Could you check a few things on this drawing? It's one solid part, dimensions in mm from its lowest x, y, z. Give positions to 0.01 mm unless a question says otherwise; leave off trailing zeros. Write each loop counter-clockwise with the first axis right and the second up, starting at its lowest first coordinate (ties: lowest second). Pieces come first, ordered by that corner, then holes. Notation, with made-up numbers: M 68.25,0.5 L 83.25,0.5 A13 cw 83.25,22.5 Z; hole C -8.75,54 d1. An arc over 180 degrees is marked long. Answer as CSV lines item,"result". Start each with the question number.
Q1. For pin 1 (8 mm diameter, centred on y = 5.5, z = 14, fed in from -X), with a flat end and sliding along its axis, tell me the tip position at first contact or that it passes through.
Q2. Suppose I cut it at A-A (z = 19). Write out the boundary of the cut face in (x, y) (1 decimal), then the cut area to 3 significant figures.
Q3. If I drill on line 1 along X through (y, z) = (37.5, 12.5); line 2 along X through (y, z) = (28.5, 12) (1 decimal); line 3 along Y through (x, z) = (16, 18.75), over which ranges is the centre line in solid material (lowest first)?
Q4. Suppose I cut it at B-B (x = 190). Write out the boundary of the cut face in (y, z).
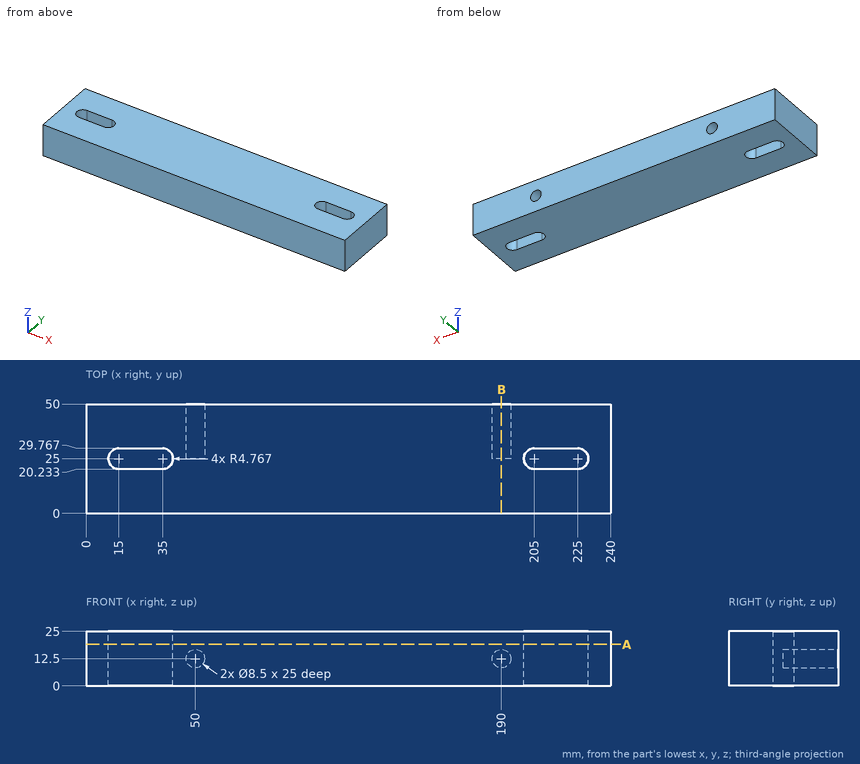
Resolved:
1,pin 1,"x = 0"
2,outline,"M 0,0 L 240,0 L 240,50 L 0,50 Z; hole M 15,20.2 L 35,20.2 A4.8 ccw 35,29.8 L 15,29.8 A4.8 ccw Z; hole M 205,20.2 L 225,20.2 A4.8 ccw 225,29.8 L 205,29.8 A4.8 ccw Z"
2,area,"11,500 mm^2"
3,line 1,"0 to 45.75, 54.25 to 185.75, 194.25 to 240"
3,line 2,"0 to 11.8, 38.2 to 45.8, 54.2 to 185.8, 194.2 to 201.8, 228.2 to 240"
3,line 3,"0 to 20.23, 29.77 to 50"
4,outline,"M 0,0 L 50,0 L 50,8.25 L 25,8.25 L 25,16.75 L 50,16.75 L 50,25 L 0,25 Z"
